Can you work these out from the drawing? Everything is in mm from the part's minimum corner. Round coordinates to 2 decimals unless told otherwise and drop trailing zeros. Order: outer loops, then holes, each group sorted by start corner. A loop starts at its lowest first (then second) coordinate and runs counter-clockwise, first axis right, second up. Notation, with made-up numbers: (11.25, 60.5) - (63.25, 60.5) arc R19 ccw to (63.25, 79.5) - close; hole circle Ø10 at (69.5, 38). An arc over 180 degrees is marked (long way). Write item = value, one per line.
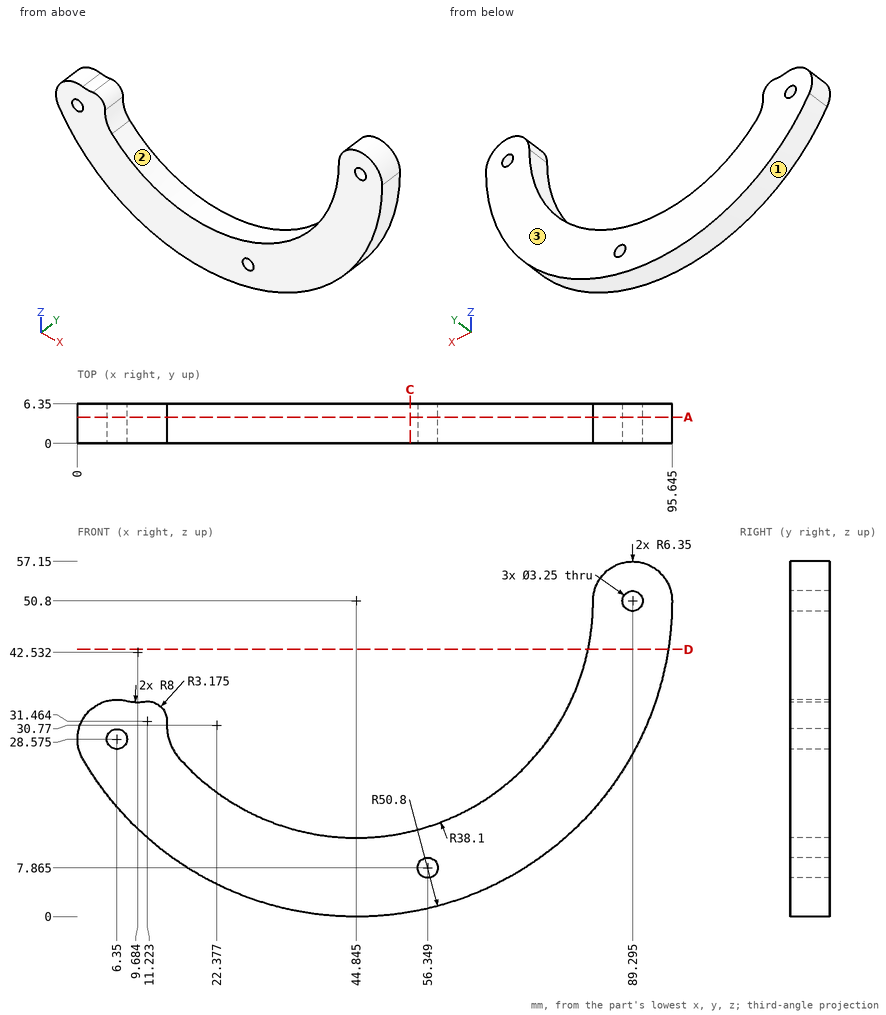
(1) If we section it at A-A (y = 4.25): State how many separate pieces and enclosed holes the cut face has, plus the area to 3 significant figures.
Computed:
separate_pieces = 1
enclosed_holes = 3
area = 1,590 mm^2
(2) If we section it at D-D (z = 43): Write out the boundary of the cut face in (x, y).
Computed:
outline = (82.14, 0) - (95.04, 0) - (95.04, 6.35) - (82.14, 6.35) - close
(3) If we section it at C-C (x = 53.5): Write out the boundary of the cut face in (y, z).
Computed:
outline = (0, 0.74) - (6.35, 0.74) - (6.35, 13.7) - (0, 13.7) - close
(4) If I drill on line 1 (X direction, y = 5, z = 50.8) (1 decimal); line 2 (X direction, y = 3.75, z = 27.5) (1 decimal); line 3 (X direction, y = 3.25, z = 21.5) (1 decimal), over which ranges is the centre line in solid material (lowest first)? Write a range as from..to.
Computed:
line_1 = 82.9..87.7, 90.9..95.6
line_2 = 0.1..5.1, 7.6..15.1, 75..90
line_3 = 3.3..20.5, 69.2..86.3
(5) Thinking about a two-plate mould opening in X: for the marked faces 1, 2 and 3, which applies, +X half, -X half, draft (parallel to the pull), parting line (faces both ways), or undercut?
Computed:
face_1 = parting line
face_2 = undercut
face_3 = draft
(6) Will these pins go through, and if not, where does the flat tip stop? P1, Ø1, axis at x = 37.5, y = 1.5, coming from the -Z side; P2, Ø1.5, axis at x = 56, y = 4, coming from the -Z side; P3, Ø2, axis at y = 3.5, z = 12.5, coming from the -X side; P4, Ø6, axis at x = 52.5, z = 10, coming from the -Y side.
Computed:
P1 = 0.46
P2 = 1.08
P3 = 10.36
P4 = 0
